CAD build for the part. Positions are in the model's coordinates, mm. A direction names the side the tool comes from. Round coordinates to 2 decimals unless told otherwise and drop trailing zeros. Write each loop counter-clockwise with the first axis right and the second up, starting at its lowest first coordinate (ties: lowest second). Pieces come first, ordered by that corner, then holes. Notation, with made-up numbers: M -20.75,2 L -12.75,2 A20 ccw -12.75,32 Z; hole C -13.5,-30 d8. An arc over 180 degrees is marked long. Write each question's results on one line, items separated by ' | '. Start each with the question number.
```python
from build123d import *

# Parameters (mm, degrees)
SKETCH1_R               = 2.075
BOSS_EXTRUDE1_DEPTH     = 4
SKETCH2_W               = 57.5
SKETCH2_H               = 9
BOSS_EXTRUDE2_DEPTH     = 5.25
CUT_EXTRUDE1_DEPTH      = 11
CUT_EXTRUDE1_DEPTH_BACK = 11
SKETCH3_W               = 10.5
SKETCH3_H               = 49.5
SKETCH4_R               = 1.55
CUT_EXTRUDE2_DEPTH      = 11


with BuildPart() as part:
    # Sketch1 → Boss-Extrude1 (new body)
    with BuildSketch(Plane(origin=(0, 0, 0), x_dir=(0, 0, -1), z_dir=(1, 0, 0))):
        with BuildLine():
            Line((0, 4.5), (65.5, 4.5))
            Line((65.5, 4.5), (65.5, -4.5))
            Line((65.5, -4.5), (0, -4.5))
            ThreePointArc((0, -4.5), (-4.5, 0), (0, 4.5))
        make_face()
        Circle(SKETCH1_R, mode=Mode.SUBTRACT)
    extrude(amount=-BOSS_EXTRUDE1_DEPTH)

    # Sketch2 → Boss-Extrude2 (add)
    with BuildSketch(Plane(origin=(0, 0, 0), x_dir=(0, 0, -1), z_dir=(1, 0, 0))):
        with Locations((36.75, 0)):
            Rectangle(SKETCH2_W, SKETCH2_H)
    extrude(amount=BOSS_EXTRUDE2_DEPTH)

    # Mirror2: part across plane


with BuildPart() as part_1:
    add(part.part)
    add(part.part.mirror(Plane(origin=(5.25, 0, 0), x_dir=(0, 0, 1), z_dir=(1, 0, 0))))

    # Sketch3 → Cut-Extrude1 (cut, two sides: drawn at the far end of the back side and taken through both)
    with BuildSketch(Plane(origin=(0, 0, 0), x_dir=(1, 0, 0), z_dir=(0, 1, 0)).offset(-CUT_EXTRUDE1_DEPTH_BACK)):
        with Locations((5.25, 36.75)):
            Rectangle(SKETCH3_W, SKETCH3_H)
    extrude(amount=CUT_EXTRUDE1_DEPTH + CUT_EXTRUDE1_DEPTH_BACK, mode=Mode.SUBTRACT)

    # Sketch4 → Cut-Extrude2 (cut)
    with BuildSketch(Plane.XY.offset(-60)):
        with Locations((5.25, 0)):
            Circle(SKETCH4_R)
    extrude(amount=-CUT_EXTRUDE2_DEPTH, mode=Mode.SUBTRACT)


solid = part_1.part
```
1) 3-axis set-ups, long thin cutter, end or side, ignore diameter. For faces 4 (the face through (3.7, 0.07, -63.47)), 5 (the face through (12.5, -0.1, 4.5)), 6 (the face through (5, -2, -61.5)), 7 (the face through (10.5, 0, -3)), 8 (the face through (12, 4.5, -32)): which of +Z, -Z, +X, -X, +Y, -Y reach the whole face in a straight line?
2) Drop a flat-ended pin along its axis: pin 1 Ø4.5 at (x, y) = (7.5, -2) entering from +Z. Give the stop position or say it passes through.
3) Saw through at C-C, the plane z = -25. Write the cut outline in (x, y).
4) Wall check: line 1 along Y through (x, z) = (5.25, -64.3); line 2 along Z through (x, y) = (6, 3.75); line 3 along Y through (x, z) = (-2.9, 0) (3 decimals). Give the ranges that are in metal, low to high. Write a range as from..to.
5) Saw through at A-A, the plane y = 0. Write the cut outline in (x, z) (3 decimals), plus the area to 3 significant figures.
6) Saw through at B-B, the plane x = 5.25. Write the cut outline in (y, z).
7) Pull direction X, two halves, no side cores. Call faces 1 (the face through (-4, 0, -31)), 2 (the face through (12.472, -2.026, 0.45)), 3 (the face through (10.5, 0, -36)): pulls with the +X half, pulls with the -X half, needs draft (parallel to the pull), parting line crosses it, or undercut.
8) Saw through at D-D, the plane x = 9.75. Write the cut outline in (y, z).
Filled sheet:
1) face 4: -Z | face 5: +Z, +X, -X | face 6: +Y, -Y | face 7: +Z, +Y, -Y | face 8: +Z, -Z, +X, -X, +Y
2) pin 1: stops at z = -8
3) outline: M -4,-4.5 L 0,-4.5 L 0,4.5 L -4,4.5 Z; M 10.5,-4.5 L 14.5,-4.5 L 14.5,4.5 L 10.5,4.5 Z
4) line 1: y = -4.5..-1.55, 1.55..4.5 | line 2: z = -65.5..-61.5, -12..-8 | line 3: y = -4.5..-2.075, 2.075..4.5
5) outline: M -4,-65.5 L 3.7,-65.5 L 3.7,-61.5 L 0,-61.5 L 0,-12 L 10.5,-12 L 10.5,-61.5 L 6.8,-61.5 L 6.8,-65.5 L 14.5,-65.5 L 14.5,-2.075 L 10.5,-2.075 L 10.5,-8 L 0,-8 L 0,-2.075 L -4,-2.075 Z; M -4,2.075 L 0,2.075 L 0,4.5 L -4,4.5 Z; M 10.5,2.075 L 14.5,2.075 L 14.5,4.5 L 10.5,4.5 Z | area: 598 mm^2
6) outline: M -4.5,-65.5 L -1.55,-65.5 L -1.55,-61.5 L -4.5,-61.5 Z; M -4.5,-12 L 4.5,-12 L 4.5,-8 L -4.5,-8 Z; M 1.55,-65.5 L 4.5,-65.5 L 4.5,-61.5 L 1.55,-61.5 Z
7) face 1: pulls with the -X half | face 2: needs draft | face 3: undercut
8) outline: M -4.5,-65.5 L 4.5,-65.5 L 4.5,-61.5 L -4.5,-61.5 Z; M -4.5,-12 L 4.5,-12 L 4.5,-8 L -4.5,-8 Z
